Verification items for the finished model (mm, model axes). Face numbers are marked on the shaded views. A direction names the side the tool comes from. Give positions to 0.01 mm unless a question says otherwise; leave off trailing zeros. Order: outer loops, then holes, each group sorted by start corner. A loop starts at its lowest first (then second) coordinate and runs counter-clockwise, first axis right, second up. Notation, with made-up numbers: (39, 27) - (93, 27) arc R12 cw to (93, 41) - close; hole circle Ø11 at (29.5, 21). An arc over 180 degrees is marked (long way). Answer as a JSON object with one key per item and string values.
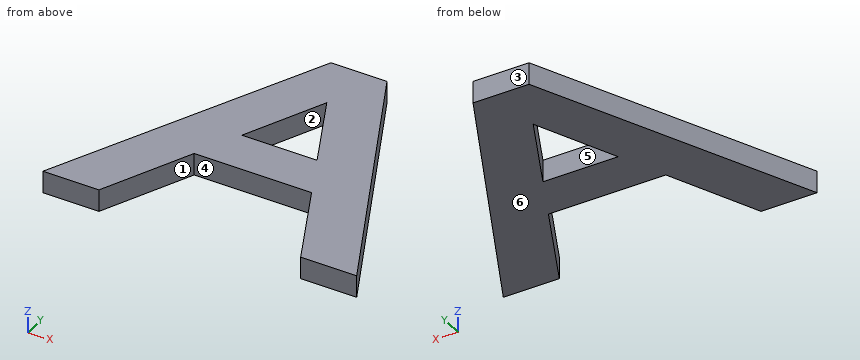
```python
from build123d import *

# Parameters (mm, degrees)
BOSS_EXTRUDE3_DEPTH = 6.35


with BuildPart() as part:
    # Sketch1 → Boss-Extrude3 (new body)
    with BuildSketch(Plane.XY):
        Polygon((0, 60.785489465), (0, 76.2), (-7.9375, 76.2), (-44.45, 0), (-28.575, 0), (-16.634568058, 25.4), (0, 25.4), (0, 38.1), (-10.664352087, 38.1), align=None)
        Polygon((7.9375, 76.2), (0, 76.2), (0, 60.785489465), (10.664352087, 38.1), (0, 38.1), (0, 25.4), (16.634568058, 25.4), (28.575, 0), (44.45, 0), align=None)
    extrude(amount=BOSS_EXTRUDE3_DEPTH)


solid = part.part
```
(1) Section check D-D (x = 30). Record the cut outline in (y, z).
Computed values:
{"outline": "(0, 0) - (30.16, 0) - (30.16, 6.35) - (0, 6.35) - close"}
(2) Release check for a two-part mould opening along Y. For the marked faces 4, 5 and 6 record: pulls with the +Y half, pulls with the -Y half, needs draft (parallel to the pull), parting line crosses it, or undercut.
Computed values:
{"face 4": "pulls with the -Y half", "face 5": "undercut", "face 6": "needs draft"}
(3) Section check B-B (y = 41). Record the cut outline in (x, z), then the cut area to 3 significant figures.
Computed values:
{"outline": "(-24.8, 0) - (-9.3, 0) - (-9.3, 6.35) - (-24.8, 6.35) - close; (9.3, 0) - (24.8, 0) - (24.8, 6.35) - (9.3, 6.35) - close", "area": "197 mm²"}
(4) Section check C-C (y = 55). Record the cut outline in (x, z), then the cut area to 3 significant figures.
Computed values:
{"outline": "(-18.1, 0) - (-2.72, 0) - (-2.72, 6.35) - (-18.1, 6.35) - close; (2.72, 0) - (18.1, 0) - (18.1, 6.35) - (2.72, 6.35) - close", "area": "195 mm²"}
(5) Gauge pin test, flat ends, axial feed: pin 1 Ø1 at (y, z) = (35, 3.5) entering from -X; pin 2 Ø2 at (y, z) = (23, 1.5) entering from +X; pin 3 Ø1 at (y, z) = (54.5, 2.5) entering from +X (3 decimals). Record the tip position at first contact, or that the pin passes through.
Computed values:
{"pin 1": "stops at x = -27.92", "pin 2": "stops at x = 33.91", "pin 3": "stops at x = 18.575"}
(6) Material ranges on line 1 along X through (y, z) = (58, 4.25); line 2 along X through (y, z) = (41.5, 3.5); line 3 along Y through (x, z) = (-7, 3.75), recorded low to high. Write a range as [from, to].
Computed values:
{"line 1": "x = [-16.66, -1.31], [1.31, 16.66]", "line 2": "x = [-24.56, -9.07], [9.07, 24.56]", "line 3": "y = [25.4, 38.1], [45.89, 76.2]"}
(7) Access from +Z, -Z, +X, -X, +Y, -Y to the whole of each face (thin tool, end or side, straight path). Record for the marked faces 1, 2 and 3.
Computed values:
{"face 1": "+Z, -Z, -Y", "face 2": "+Z, -Z", "face 3": "+Z, -Z, +X, -X, +Y"}
